```python
from build123d import *

# Parameters (mm, degrees)
M2_SCREW_SHANK_PROFILE_R  = 1
M2_SCREW_SHANK_DEPTH      = 16
SOCKET_CAP_HEAD_PROFILE_R = 1.9
SOCKET_CAP_HEAD_DEPTH     = 2
CUT_HEX_KEY_RECESS_DEPTH  = 1.2


with BuildPart() as part:
    # M2 screw shank profile → M2 screw shank (new body)
    with BuildSketch(Plane.XY.offset(3.2)):
        with Locations((-63.291651246, -5.5)):
            Circle(M2_SCREW_SHANK_PROFILE_R)
    extrude(amount=M2_SCREW_SHANK_DEPTH)

    # Socket cap head profile → Socket cap head (add)
    with BuildSketch(Plane.XY.offset(19.2)):
        with Locations((-63.291651246, -5.5)):
            Circle(SOCKET_CAP_HEAD_PROFILE_R)
    extrude(amount=SOCKET_CAP_HEAD_DEPTH)

    # Hex key socket → Cut hex key recess (cut)
    with BuildSketch(Plane.XY.offset(20.1)):
        Polygon((-62.541651246, -5.066987298), (-63.291651246, -4.633974596), (-64.041651246, -5.066987298), (-64.041651246, -5.933012702), (-63.291651246, -6.366025404), (-62.541651246, -5.933012702), align=None)
    extrude(amount=CUT_HEX_KEY_RECESS_DEPTH, mode=Mode.SUBTRACT)


solid = part.part
```
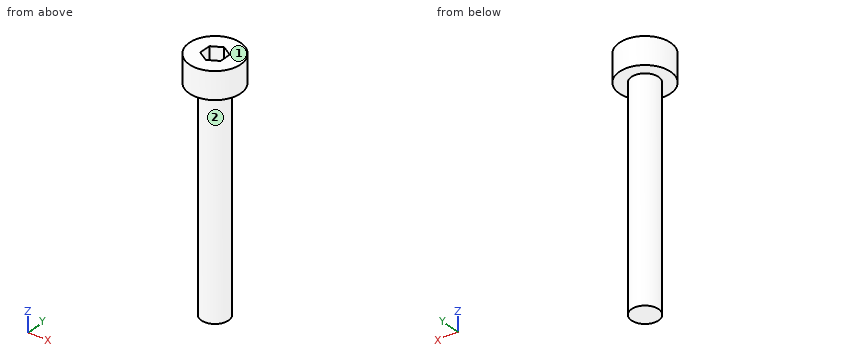
Geometry: final body of the model. Coordinates: model frame, mm. Face numbers are marked on the shaded views. A direction names the side the tool comes from. Round coordinates to 2 decimals unless told otherwise and drop trailing zeros. Order: outer loops, then holes, each group sorted by start corner. A loop starts at its lowest first (then second) coordinate and runs counter-clockwise, first axis right, second up. Notation, with made-up numbers: (-11.5, 44) - (44.5, 44) arc R15 cw to (44.5, 54) - close; hole circle Ø7 at (64.25, -11). An arc over 180 degrees is marked (long way). Use CSV: the item, a comma, the result in double quotes. Start each with the question number.
Q1. Material intervals for line 1 along Z through (x, y) = (-62.7, -4.6); line 2 along X through (y, z) = (-5.45, 8.25); line 3 along X through (y, z) = (-5.85, 20.75), sorted ascending. Write a range as from..to.
Q2. First-contact query: pin 1 (1.6 mm diameter, centred on x = -63.5, y = -5.5, fed in from +Z); pin 2 (2 mm diameter, centred on x = -64.5, z = 15, fed in from +Y). Flat tips, straight axial feed; report the tip coordinate or a pass-through.
Q3. Section query B-B (y = -5.5). Return loops of the section in (x, z), and give its area (4 significant figures).
Q4. Section query C-C (z = 9.5). Return loops of the section in (x, y), and give its area (3 significant figures).
Q5. Access query for the marked faces 1 and 2. Directions: +Z, -Z, +X, -X, +Y, -Y. A direction counts if a zero-diameter tool reaches every point of the face in a straight line with its end or side. Return the directions, or none.
Q6. Section query A-A (x = -62.7). Return loops of the section in (y, z).
Q7. Section query D-D (x = -61.95). Return loops of the section in (y, z).
Result set:
1,line 1,"z = 19.2..21.2"
1,line 2,"x = -64.29..-62.29"
1,line 3,"x = -65.16..-64.04, -62.54..-61.42"
2,pin 1,"stops at z = 21.2"
2,pin 2,"stops at y = -4.52"
3,outline,"(-65.19, 19.2) - (-64.29, 19.2) - (-64.29, 3.2) - (-62.29, 3.2) - (-62.29, 19.2) - (-61.39, 19.2) - (-61.39, 21.2) - (-62.54, 21.2) - (-62.54, 20.1) - (-64.04, 20.1) - (-64.04, 21.2) - (-65.19, 21.2) - close"
3,area,"37.95 mm2"
4,outline,"circle Ø2 at (-63.29, -5.5)"
4,area,"3.14 mm2"
5,face 1,"+Z, +X, -X, +Y, -Y"
5,face 2,"-Z"
6,outline,"(-7.31, 19.2) - (-6.31, 19.2) - (-6.31, 3.2) - (-4.69, 3.2) - (-4.69, 19.2) - (-3.69, 19.2) - (-3.69, 21.2) - (-4.98, 21.2) - (-4.98, 20.1) - (-6.02, 20.1) - (-6.02, 21.2) - (-7.31, 21.2) - close"
7,outline,"(-6.85, 19.2) - (-4.15, 19.2) - (-4.15, 21.2) - (-6.85, 21.2) - close"
